```python
from build123d import *

# Parameters (mm, degrees)
SKETCH_R     = 1.8
SKETCH_R_2   = 3.9
SKETCH_R_3   = 1.1
PAD_DEPTH    = 2
SKETCH001_W  = 2
SKETCH001_H  = 42
PAD001_DEPTH = 2
POCKET_DEPTH = 4.001


with BuildPart() as part:
    # Sketch → Pad (new body)
    with BuildSketch(Plane.XY):
        Polygon((-8, 42), (3, 42), (3, 12), (0, 12), (0, 0), (-8, 0), align=None)
        with Locations((-3, 3)):
            Circle(SKETCH_R, mode=Mode.SUBTRACT)
        with Locations((-2, 36)):
            Circle(SKETCH_R_2, mode=Mode.SUBTRACT)
        with Locations((-2, 22)):
            Circle(SKETCH_R_3, mode=Mode.SUBTRACT)
    extrude(amount=PAD_DEPTH)

    # Sketch001 → Pad001 (new body)
    with BuildSketch(Plane.XY.offset(2)):
        with Locations((-7, 21)):
            Rectangle(SKETCH001_W, SKETCH001_H)
    extrude(amount=PAD001_DEPTH)

    # Sketch002 → Pocket (cut, through all)
    with BuildSketch(Plane.XY.offset(4)):
        with BuildLine():
            ThreePointArc((-2.000021, 42), (-6.242641, 40.242641), (-8, 36.000021))
            Line((-8, 36.000021), (-8, 42))
            Line((-8, 42), (-2.000021, 42))
        make_face()
    extrude(amount=-POCKET_DEPTH, mode=Mode.SUBTRACT)


solid = part.part
```
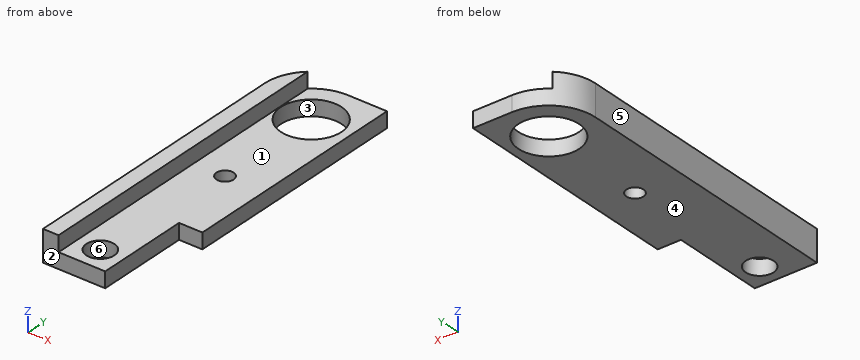
Here's how the part is built. I have some questions about the finished solid (model axes, mm). Face numbers are marked on the shaded views. A direction names the side the tool comes from. Give positions to 0.01 mm unless a question says otherwise; leave off trailing zeros. Write each loop counter-clockwise with the first axis right and the second up, starting at its lowest first coordinate (ties: lowest second). Pieces come first, ordered by that corner, then holes. Notation, with made-up numbers: (23, 23) -> (60, 23) arc R27 ccw to (60, 40) -> close; hole circle Ø9 at (-9, 26). An arc over 180 degrees is marked (long way). Use one line per item in the form item = value.
1) Suppose I cut it at C-C (x = -4.25). Please give me the cut outline in (y, z), and give its area (3 significant figures).
Verdict:
outline = (0, 0) -> (1.7, 0) -> (1.7, 2) -> (0, 2) -> close; (4.3, 0) -> (32.81, 0) -> (32.81, 2) -> (4.3, 2) -> close; (39.19, 0) -> (41.56, 0) -> (41.56, 2) -> (39.19, 2) -> close
area = 65.2 mm2
2) I'm going to push flat-ended pins straight in: pin 1 (1.6 mm diameter, centred on x = 2, z = 1, fed in from -Y); pin 2 (0.6 mm diameter, centred on y = 20.5, z = 3, fed in from +X); pin 3 (6 mm diameter, centred on x = -2.5, y = 35, fed in from +Z). Where does each tip first touch, or does it pass through?
Verdict:
pin_1 = 12
pin_2 = -6
pin_3 = 2
3) Suppose I cut it at A-A (y = 22). Please give me the cut outline in (x, z).
Verdict:
outline = (-8, 0) -> (-3.1, 0) -> (-3.1, 2) -> (-6, 2) -> (-6, 4) -> (-8, 4) -> close; (-0.9, 0) -> (3, 0) -> (3, 2) -> (-0.9, 2) -> close
4) If I drill on L1, parallel to Y at x = -3, z = 1.5; L2, parallel to Y at x = -2, z = 0.8; L3, parallel to Z at x = 2.5, y = 19.5, over which ranges is the centre line in solid material (lowest first)? Write a range as [from, to].
Verdict:
L1 = [0, 1.2], [4.8, 21.54], [22.46, 32.23], [39.77, 41.92]
L2 = [0, 1.5], [4.5, 20.9], [23.1, 32.1], [39.9, 42]
L3 = [0, 2]
5) On a 3-axis mill with a long thin cutter (end or side, diameter ignored), from which of +Z, -Z, +X, -X, +Y, -Y can I reach the whole of each face in a straight line? I mean the marked faces 1 and 2. Say none if no direction works.
Verdict:
face_1 = +Z, +X, +Y, -Y
face_2 = +Z, -Z, +X, -X, -Y
6) We'd pull the mould along X, two halves only. Please class the marked faces 3, 4, 5 and 6: +X half, -X half, draft (parallel to the pull), parting line (faces both ways), or undercut.
Verdict:
face_3 = undercut
face_4 = draft
face_5 = -X half
face_6 = undercut
7) Suppose I cut it at D-D (y = 12.5). Please give me the cut outline in (x, z).
Verdict:
outline = (-8, 0) -> (3, 0) -> (3, 2) -> (-6, 2) -> (-6, 4) -> (-8, 4) -> close
8) Suppose I cut it at B-B (x = -0.5). Please give me the cut outline in (y, z).
Verdict:
outline = (0, 0) -> (32.4, 0) -> (32.4, 2) -> (0, 2) -> close; (39.6, 0) -> (42, 0) -> (42, 2) -> (39.6, 2) -> close
